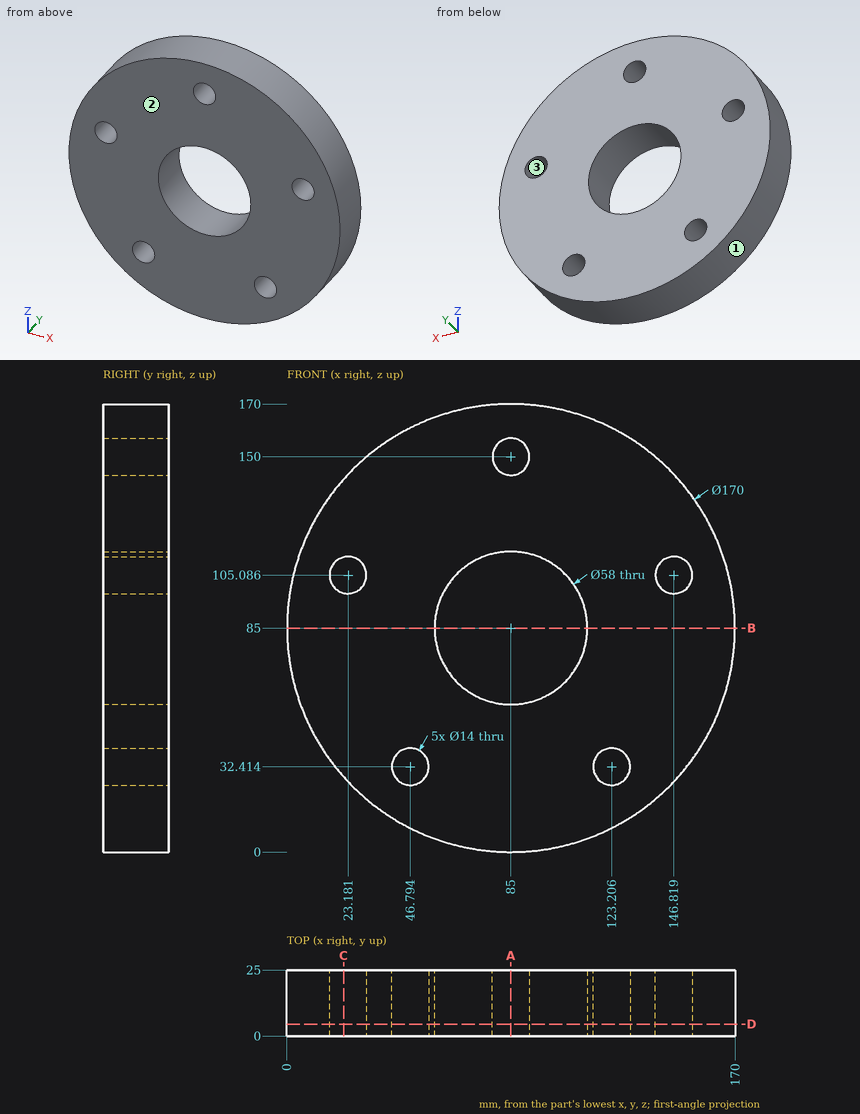
Study the drawing (mm; zero at the part's minimum x, y, z) and answer. Give positions to 0.01 mm unless a question says otherwise; leave off trailing zeros. Loops run counter-clockwise (first coordinate to the right, second up) from the corner with the lowest first, then second, coordinate; pieces in that order, holes last. Notation, with made-up numbers: (41, -40) - (65, -40) arc R36 ccw to (65, -3) - close; hole circle Ø2 at (84, 33.5). An arc over 180 degrees is marked (long way). Answer in a Markdown table with one row per item. Add a question column.
Q1. Determine the mould class of the marked faces 1, 2 and 3 for opening direction X: released by +X, released by -X, zero draft, split by the parting line, or undercut.
Q2. The part is cut by section B-B (z = 85). Determine the outline of the cut face in (x, y), and give its area (3 significant figures).
Q3. Each of these flat-tipped pins is pushed along its axis until it touches: P1, Ø12, axis at y = 4.5, z = 138, coming from the +X side; P2, Ø2, axis at x = 62, y = 11.5, coming from the -Z side; P3, Ø1, axis at y = 19, z = 26, coming from the +X side; P4, Ø8.5, axis at x = 146.82, z = 105.09, coming from the +Y side. Where does it stop, or does it pass through?
Q4. The part is cut by section C-C (x = 21.5). Determine the outline of the cut face in (y, z) (1 decimal), and give its area (3 significant figures).
Q5. Consider line 1 along Z through (x, y) = (85, 10); line 2 along X through (y, z) = (23.5, 31); line 3 along Z through (x, y) = (141.5, 20) (1 decimal). Determine where each line is inside the solid, lowest interval first.
Q6. The part is cut by section D-D (y = 4.5). Determine the outline of the cut face in (x, z).
Q7. The part is cut by section A-A (x = 85). Determine the outline of the cut face in (y, z), and give its area (3 significant figures).
Solution:
| question | item | result |
|---|---|---|
| 1 | face 1 | split by the parting line |
| 1 | face 2 | zero draft |
| 1 | face 3 | undercut |
| 2 | outline | (0, 0) - (56, 0) - (56, 25) - (0, 25) - close; (114, 0) - (170, 0) - (170, 25) - (114, 25) - close |
| 2 | area | 2,800 mm² |
| 3 | P1 | stops at x = 155.82 |
| 3 | P2 | stops at z = 2.9 |
| 3 | P3 | stops at x = 146.67 |
| 3 | P4 | passes through |
| 4 | outline | (0, 28.5) - (25, 28.5) - (25, 98.3) - (0, 98.3) - close; (0, 111.9) - (25, 111.9) - (25, 141.5) - (0, 141.5) - close |
| 4 | area | 2,490 mm² |
| 5 | line 1 | z = 0 to 56, 114 to 143, 157 to 170 |
| 5 | line 2 | x = 19.36 to 39.94, 53.65 to 116.35, 130.06 to 150.64 |
| 5 | line 3 | z = 21.5 to 100.5, 109.6 to 148.5 |
| 6 | outline | circle Ø170 at (85, 85); hole circle Ø14 at (23.18, 105.09); hole circle Ø14 at (46.79, 32.41); hole circle Ø58 at (85, 85); hole circle Ø14 at (85, 150); hole circle Ø14 at (123.21, 32.41); hole circle Ø14 at (146.82, 105.09) |
| 7 | outline | (0, 0) - (25, 0) - (25, 56) - (0, 56) - close; (0, 114) - (25, 114) - (25, 143) - (0, 143) - close; (0, 157) - (25, 157) - (25, 170) - (0, 170) - close |
| 7 | area | 2,450 mm² |
